```python
from build123d import *

# Parameters (mm, degrees)
F0_R     = 3.175
F1_DEPTH = 3.048
F2_DEPTH = 50.8


with BuildPart() as f1:
    # F0 (on Front) → F1 (new body)
    with BuildSketch(Plane.XZ):
        with BuildLine():
            Line((15.7474569047, 65.5082893304), (9.525, 114.3))
            ThreePointArc((9.525, 114.3), (0, 104.775), (-9.525, 114.3))
            Line((-9.525, 114.3), (-15.7474569047, 65.5082893304))
            ThreePointArc((-15.7474569047, 65.5082893304), (0, 79.375), (15.7474569047, 65.5082893304))
        make_face()
        with Locations((3.175, 100.0252)):
            Circle(F0_R, mode=Mode.SUBTRACT)
        with BuildLine():
            ThreePointArc((-9.525, 114.3), (0, 104.775), (9.525, 114.3))
            ThreePointArc((9.525, 114.3), (0, 123.825), (-9.525, 114.3))
        make_face()
        with Locations((0, 114.3)):
            Circle(F0_R, mode=Mode.SUBTRACT)
        with BuildLine():
            ThreePointArc((15.875, 63.5), (15.8430821396, 64.5061676396), (15.7474569047, 65.5082893304))
            ThreePointArc((15.7474569047, 65.5082893304), (0, 79.375), (-15.7474569047, 65.5082893304))
            ThreePointArc((-15.7474569047, 65.5082893304), (-15.8735876171, 63.7117573215), (-15.7954255641, 61.9125))
            ThreePointArc((-15.7954255641, 61.9125), (-0.0060905531, 47.6250011683), (15.7942028036, 61.9003804205))
            ThreePointArc((15.7942028036, 61.9003804205), (15.8547878338, 62.6991705884), (15.875, 63.5))
        make_face()
        with Locations((0, 63.5)):
            Circle(F0_R, mode=Mode.SUBTRACT)
        with BuildLine():
            ThreePointArc((15.7942028036, 61.9003804205), (-0.0060905531, 47.6250011683), (-15.7954255641, 61.9125))
            Line((-15.7954255641, 61.9125), (-11.3411865923, 17.5933818124))
            ThreePointArc((-11.3411865923, 17.5933818124), (-13.2611998974, 11.5713591498), (-18.9676000005, 8.8532337108))
            Line((-18.9676000005, 8.8532337108), (-44.7334821429, 7.9324362036))
            ThreePointArc((-44.7334821429, 7.9324362036), (-38.9384772185, 5.7120069047), (-36.5125, 0))
            ThreePointArc((-36.5125, 0), (-38.9380895153, -5.7116327839), (-44.7324052746, -7.9324746146))
            Line((-44.7324052746, -7.9324746146), (-0.6773435479, -9.500885786))
            ThreePointArc((-0.6773435479, -9.500885786), (-6.4912990883, 6.9705567315), (9.525, 0))
            Line((9.525, 0), (15.7942028036, 61.9003804205))
        make_face()
        with BuildLine():
            ThreePointArc((0, -9.525), (6.7351920908, -6.7351920908), (9.525, 0))
            ThreePointArc((9.525, 0), (-6.4912990883, 6.9705567315), (-0.6773435479, -9.500885786))
            Line((-0.6773435479, -9.500885786), (0, -9.525))
        make_face()
        Circle(F0_R, mode=Mode.SUBTRACT)
        with BuildLine():
            ThreePointArc((-36.5125, 0), (-38.9384772185, 5.7120069047), (-44.7334821429, 7.9324362036))
            ThreePointArc((-44.7334821429, 7.9324362036), (-52.3874999817, -0.0005387766), (-44.7324052746, -7.9324746146))
            ThreePointArc((-44.7324052746, -7.9324746146), (-38.9380895153, -5.7116327839), (-36.5125, 0))
        make_face()
        with Locations((-44.45, 0)):
            Circle(F0_R, mode=Mode.SUBTRACT)
    extrude(amount=F1_DEPTH)

    # F2 (add): a face of the model
    f2_faces = [f1.faces().sort_by_distance(p)[0] for p in [
        (-5.2061235435, 0, 46.6226606697),
    ]]
    extrude(f2_faces, amount=F2_DEPTH)


solid = f1.part
```
Geometry: final body of the model. Coordinates: model frame, mm. A direction names the side the tool comes from. Round coordinates to 2 decimals unless told otherwise and drop trailing zeros. Order: outer loops, then holes, each group sorted by start corner. A loop starts at its lowest first (then second) coordinate and runs counter-clockwise, first axis right, second up. Notation, with made-up numbers: (32.5, 87) -> (69.5, 87) arc R26 cw to (69.5, 119) -> close; hole circle Ø10 at (-11.5, 29.25). An arc over 180 degrees is marked (long way). Write each question's results on one line, items separated by ' | '.
Q1. Pull-direction query (Z, two-part tool) for faces 3 (the face through (12.616, 23.499, 30.517)), 4 (the face through (-13.2, 23.5, 11.64)), 5 (the face through (-4, 50.8, 43)); classes: released by +Z, released by -Z, zero draft, split by the parting line, or undercut.
Response values:
face 3: released by -Z | face 4: undercut | face 5: zero draft
Q2. Section query C-C (x = -8). Output: boundary loops of the cut face in (y, z), and give its area (3 significant figures).
Response values:
outline: (-3.05, -9.24) -> (50.8, -9.24) -> (50.8, 119.47) -> (-3.05, 119.47) -> close | area: 6,930 mm²
Q3. Ray query, line 1 along Z through (x, y) = (-1, 11); line 2 along Z through (x, y) = (-0.5, 25); line 3 along Z through (x, y) = (-44.5, 42). Return the intervals inside material, ascending.
Response values:
line 1: -9.49 to -3.01, 3.01 to 60.49, 66.51 to 111.29, 117.31 to 123.77 | line 2: -9.51 to -3.14, 3.14 to 60.36, 66.64 to 111.16, 117.44 to 123.81 | line 3: -7.94 to -3.17, 3.17 to 7.94
Q4. Pin query (flat end, axial travel): pin 1 Ø12 at (y, z) = (8.5, 44) entering from +X; pin 2 Ø5 at (x, z) = (0, 63.5) entering from -Y; pin 3 Ø10 at (y, z) = (8.5, 27) entering from +X; pin 4 Ø1 at (y, z) = (30, 53) entering from +X. Return the tip coordinate at first contact, or that it passes through.
Response values:
pin 1: x = 14.59 | pin 2: through | pin 3: x = 12.77 | pin 4: x = 14.94
Q5. Section query A-A (y = 39.5). Count the separate pieces of the cut face and the enclosed holes in it, and give its area (3 significant figures).
Response values:
separate pieces: 1 | enclosed holes: 5 | area: 3,770 mm²
Q6. Access query for faces 1 (the face through (6.66, 23.5, -6.81)), 2 (the face through (-13.6, 23.5, 40.06)). Directions: +Z, -Z, +X, -X, +Y, -Y. A direction counts if a zero-diameter tool reaches every point of the face in a straight line with its end or side. Return the directions, or none.
Response values:
face 1: -Z, +X, +Y, -Y | face 2: -X, +Y, -Y
Q7. Section query B-B (z = 75.5). Output: boundary loops of the cut face in (x, y).
Response values:
outline: (-14.47, -3.05) -> (14.47, -3.05) -> (14.47, 50.8) -> (-14.47, 50.8) -> close
